Verification items for the finished model (mm, model axes). Coordinates: 2 decimals unless noted, no trailing zeros. Order: outer loops, then holes, each group sorted by start corner. A loop starts at its lowest first (then second) coordinate and runs counter-clockwise, first axis right, second up. Notation, with made-up numbers: (-16.75, 88.5) -> (-7.75, 88.5) arc R10 cw to (-7.75, 102.5) -> close; hole circle Ø6 at (-28, 72). An arc over 180 degrees is marked (long way). Write item = value, one per line. Start each with the question number.
from build123d import *

# Parameters (mm, degrees)
F0_W     = 254
F0_H     = 330.2
F1_DEPTH = 3.175
F3_DEPTH = 3.175
F4_R     = 60
F5_DEPTH = 3.175


with BuildPart() as f1:
    # F0 (on Front) → F1 (new body)
    with BuildSketch(Plane.XZ):
        with Locations((-49.04184, 40.386009)):
            Rectangle(F0_W, F0_H)
    extrude(amount=F1_DEPTH)

    # F2 (on face) → F3 (cut, through all)
    with BuildSketch(Plane.XZ.offset(3.175)):
        with BuildLine():
            ThreePointArc((68.25536, 173.240709), (68.344315, 173.242267), (68.43316, 173.24694))
            Line((68.43316, 173.24694), (68.43316, 189.109479))
            ThreePointArc((68.43316, 189.109479), (68.344315, 189.114151), (68.25536, 189.115709))
            Line((68.25536, 189.115709), (-20.33984, 189.115709))
            ThreePointArc((-20.33984, 189.115709), (-22.135891, 188.371761), (-22.87984, 186.575709))
            Line((-22.87984, 186.575709), (-22.87984, 175.780709))
            ThreePointArc((-22.87984, 175.780709), (-22.135891, 173.984658), (-20.33984, 173.240709))
            Line((-20.33984, 173.240709), (68.25536, 173.240709))
        make_face()
        with BuildLine():
            Line((68.43316, 189.109479), (68.43316, 173.24694))
            ThreePointArc((68.43316, 173.24694), (70.11321, 174.04866), (70.79536, 175.780709))
            Line((70.79536, 175.780709), (70.79536, 186.575709))
            ThreePointArc((70.79536, 186.575709), (70.11321, 188.307758), (68.43316, 189.109479))
        make_face()
        with BuildLine():
            ThreePointArc((68.25536, 152.920709), (68.344315, 152.922267), (68.43316, 152.92694))
            Line((68.43316, 152.92694), (68.43316, 168.789479))
            ThreePointArc((68.43316, 168.789479), (68.344315, 168.794151), (68.25536, 168.795709))
            Line((68.25536, 168.795709), (-20.33984, 168.795709))
            ThreePointArc((-20.33984, 168.795709), (-22.135891, 168.051761), (-22.87984, 166.255709))
            Line((-22.87984, 166.255709), (-22.87984, 155.460709))
            ThreePointArc((-22.87984, 155.460709), (-22.135891, 153.664658), (-20.33984, 152.920709))
            Line((-20.33984, 152.920709), (68.25536, 152.920709))
        make_face()
        with BuildLine():
            Line((68.43316, 168.789479), (68.43316, 152.92694))
            ThreePointArc((68.43316, 152.92694), (70.11321, 153.72866), (70.79536, 155.460709))
            Line((70.79536, 155.460709), (70.79536, 166.255709))
            ThreePointArc((70.79536, 166.255709), (70.11321, 167.987758), (68.43316, 168.789479))
        make_face()
        with BuildLine():
            ThreePointArc((68.25536, 132.600709), (68.344315, 132.602267), (68.43316, 132.60694))
            Line((68.43316, 132.60694), (68.43316, 148.469479))
            ThreePointArc((68.43316, 148.469479), (68.344315, 148.474151), (68.25536, 148.475709))
            Line((68.25536, 148.475709), (-20.33984, 148.475709))
            ThreePointArc((-20.33984, 148.475709), (-22.135891, 147.731761), (-22.87984, 145.935709))
            Line((-22.87984, 145.935709), (-22.87984, 135.140709))
            ThreePointArc((-22.87984, 135.140709), (-22.135891, 133.344658), (-20.33984, 132.600709))
            Line((-20.33984, 132.600709), (68.25536, 132.600709))
        make_face()
        with BuildLine():
            Line((68.43316, 148.469479), (68.43316, 132.60694))
            ThreePointArc((68.43316, 132.60694), (70.11321, 133.40866), (70.79536, 135.140709))
            Line((70.79536, 135.140709), (70.79536, 145.935709))
            ThreePointArc((70.79536, 145.935709), (70.11321, 147.667758), (68.43316, 148.469479))
        make_face()
        with BuildLine():
            ThreePointArc((68.25536, 112.280709), (68.344315, 112.282267), (68.43316, 112.28694))
            Line((68.43316, 112.28694), (68.43316, 128.149479))
            ThreePointArc((68.43316, 128.149479), (68.344315, 128.154151), (68.25536, 128.155709))
            Line((68.25536, 128.155709), (-20.33984, 128.155709))
            ThreePointArc((-20.33984, 128.155709), (-22.135891, 127.411761), (-22.87984, 125.615709))
            Line((-22.87984, 125.615709), (-22.87984, 114.820709))
            ThreePointArc((-22.87984, 114.820709), (-22.135891, 113.024658), (-20.33984, 112.280709))
            Line((-20.33984, 112.280709), (68.25536, 112.280709))
        make_face()
        with BuildLine():
            Line((68.43316, 128.149479), (68.43316, 112.28694))
            ThreePointArc((68.43316, 112.28694), (70.11321, 113.08866), (70.79536, 114.820709))
            Line((70.79536, 114.820709), (70.79536, 125.615709))
            ThreePointArc((70.79536, 125.615709), (70.11321, 127.347758), (68.43316, 128.149479))
        make_face()
        with BuildLine():
            ThreePointArc((68.25536, 91.960709), (68.344315, 91.962267), (68.43316, 91.96694))
            Line((68.43316, 91.96694), (68.43316, 107.829479))
            ThreePointArc((68.43316, 107.829479), (68.344315, 107.834151), (68.25536, 107.835709))
            Line((68.25536, 107.835709), (-20.33984, 107.835709))
            ThreePointArc((-20.33984, 107.835709), (-22.135891, 107.091761), (-22.87984, 105.295709))
            Line((-22.87984, 105.295709), (-22.87984, 94.500709))
            ThreePointArc((-22.87984, 94.500709), (-22.135891, 92.704658), (-20.33984, 91.960709))
            Line((-20.33984, 91.960709), (68.25536, 91.960709))
        make_face()
        with BuildLine():
            Line((68.43316, 107.829479), (68.43316, 91.96694))
            ThreePointArc((68.43316, 91.96694), (70.11321, 92.76866), (70.79536, 94.500709))
            Line((70.79536, 94.500709), (70.79536, 105.295709))
            ThreePointArc((70.79536, 105.295709), (70.11321, 107.027758), (68.43316, 107.829479))
        make_face()
        with BuildLine():
            ThreePointArc((68.25536, 71.640709), (68.344315, 71.642267), (68.43316, 71.64694))
            Line((68.43316, 71.64694), (68.43316, 87.509479))
            ThreePointArc((68.43316, 87.509479), (68.344315, 87.514151), (68.25536, 87.515709))
            Line((68.25536, 87.515709), (-20.33984, 87.515709))
            ThreePointArc((-20.33984, 87.515709), (-22.135891, 86.771761), (-22.87984, 84.975709))
            Line((-22.87984, 84.975709), (-22.87984, 74.180709))
            ThreePointArc((-22.87984, 74.180709), (-22.135891, 72.384658), (-20.33984, 71.640709))
            Line((-20.33984, 71.640709), (68.25536, 71.640709))
        make_face()
        with BuildLine():
            Line((68.43316, 87.509479), (68.43316, 71.64694))
            ThreePointArc((68.43316, 71.64694), (70.11321, 72.44866), (70.79536, 74.180709))
            Line((70.79536, 74.180709), (70.79536, 84.975709))
            ThreePointArc((70.79536, 84.975709), (70.11321, 86.707758), (68.43316, 87.509479))
        make_face()
        with BuildLine():
            ThreePointArc((68.25536, 51.320709), (68.344315, 51.322267), (68.43316, 51.32694))
            Line((68.43316, 51.32694), (68.43316, 67.189479))
            ThreePointArc((68.43316, 67.189479), (68.344315, 67.194151), (68.25536, 67.195709))
            Line((68.25536, 67.195709), (-20.33984, 67.195709))
            ThreePointArc((-20.33984, 67.195709), (-22.135891, 66.451761), (-22.87984, 64.655709))
            Line((-22.87984, 64.655709), (-22.87984, 53.860709))
            ThreePointArc((-22.87984, 53.860709), (-22.135891, 52.064658), (-20.33984, 51.320709))
            Line((-20.33984, 51.320709), (68.25536, 51.320709))
        make_face()
        with BuildLine():
            Line((68.43316, 67.189479), (68.43316, 51.32694))
            ThreePointArc((68.43316, 51.32694), (70.11321, 52.12866), (70.79536, 53.860709))
            Line((70.79536, 53.860709), (70.79536, 64.655709))
            ThreePointArc((70.79536, 64.655709), (70.11321, 66.387758), (68.43316, 67.189479))
        make_face()
        with BuildLine():
            Line((68.25536, 46.990009), (28.63136, 46.990009))
            ThreePointArc((28.63136, 46.990009), (26.835309, 46.246061), (26.09136, 44.450009))
            Line((26.09136, 44.450009), (26.09136, -109.473991))
            ThreePointArc((26.09136, -109.473991), (26.835309, -111.270042), (28.63136, -112.013991))
            Line((28.63136, -112.013991), (68.25536, -112.013991))
            ThreePointArc((68.25536, -112.013991), (70.051412, -111.270042), (70.79536, -109.473991))
            Line((70.79536, -109.473991), (70.79536, 44.450009))
            ThreePointArc((70.79536, 44.450009), (70.11321, 46.182058), (68.43316, 46.983779))
            ThreePointArc((68.43316, 46.983779), (68.344315, 46.988451), (68.25536, 46.990009))
        make_face()
    extrude(amount=-F3_DEPTH, mode=Mode.SUBTRACT)

    # F4 (on face) → F5 (cut, through all)
    with BuildSketch(Plane.XZ.offset(3.175)):
        with Locations((-50.10864, -32.638991)):
            Circle(F4_R)
    extrude(amount=-F5_DEPTH, mode=Mode.SUBTRACT)


solid = f1.part
Item 1: Mould release check, pull along X, two halves, no side actions. Record for faces 1 (the flat face through (-79, -3.175, 79)), 2 (the cylindrical face through (-63.12, -1.61, -91.21)): pulls with the +X half, pulls with the -X half, needs draft (parallel to the pull), parting line crosses it, or undercut.
Item 2: Thickness scan on line 1 (X direction, y = -2.55, z = 64.5); line 2 (X direction, y = -2.05, z = -62); line 3 (X direction, y = -0.5, z = -67). Record the ranges inside material, lowest first.
Item 3: Section check A-A (z = 162). Record the boundary of the cut face in (x, y) (3 decimals).
Item 4: Section check D-D (z = 4). Record the boundary of the cut face in (x, y) (3 decimals), then the cut area to 3 significant figures.
Item 5: Section check C-C (z = -41.5). Record the boundary of the cut face in (x, y) (3 decimals).
Item 6: Section check B-B (x = -84). Record the boundary of the cut face in (y, z) (3 decimals).
Filled sheet:
q1.face_1 = needs draft
q1.face_2 = undercut
q2.line_1 = -176.04 to -22.88, 70.8 to 77.96
q2.line_2 = -176.04 to -102.43, 2.22 to 26.09, 70.8 to 77.96
q2.line_3 = -176.04 to -99.3, -0.92 to 26.09, 70.8 to 77.96
q3.outline = (-176.042, -3.175) -> (-22.88, -3.175) -> (-22.88, 0) -> (-176.042, 0) -> close; (70.795, -3.175) -> (77.958, -3.175) -> (77.958, 0) -> (70.795, 0) -> close
q4.outline = (-176.042, -3.175) -> (-97.623, -3.175) -> (-97.623, 0) -> (-176.042, 0) -> close; (-2.595, -3.175) -> (26.091, -3.175) -> (26.091, 0) -> (-2.595, 0) -> close; (70.795, -3.175) -> (77.958, -3.175) -> (77.958, 0) -> (70.795, 0) -> close
q4.area = 363 mm^2
q5.outline = (-176.042, -3.175) -> (-109.451, -3.175) -> (-109.451, 0) -> (-176.042, 0) -> close; (9.233, -3.175) -> (26.091, -3.175) -> (26.091, 0) -> (9.233, 0) -> close; (70.795, -3.175) -> (77.958, -3.175) -> (77.958, 0) -> (70.795, 0) -> close
q6.outline = (-3.175, -124.714) -> (0, -124.714) -> (0, -82.15) -> (-3.175, -82.15) -> close; (-3.175, 16.872) -> (0, 16.872) -> (0, 205.486) -> (-3.175, 205.486) -> close
